Part model, mm, in its own coordinate system. Face numbers are marked on the shaded views. A direction names the side the tool comes from. Round coordinates to 2 decimals unless told otherwise and drop trailing zeros. Order: outer loops, then holes, each group sorted by start corner. A loop starts at its lowest first (then second) coordinate and runs counter-clockwise, first axis right, second up. Notation, with made-up numbers: (61.25, 66.5) - (87.25, 66.5) arc R16 cw to (87.25, 72.5) - close; hole circle Ø8 at (56.25, 64.25). An arc over 180 degrees is marked (long way). Return JSON: item names as keys, results as strings. Group by question number.
Item 1: Saw through at A-A on z = 37.5. List the corners of the cut face in (x, y) (3 decimals).
Item 2: Tool access for the marked faces 1, 2 and 3: list every direction of +Z, -Z, +X, -X, +Y, -Y with a clear straight run to the whole face (end or side of a thin tool).
Item 3: Saw through at D-D on z = 26. List the corners of the cut face in (x, y) (3 decimals), and give its area (3 significant figures).
Item 4: Probe probe 1 along X at (y, z) = (-53, 14.5) (3 decimals); probe 2 along Y at (x, z) = (20, 4.5) (3 decimals); probe 3 along Z at (x, y) = (-15, -66). List the from-to ranges inside material, lowest first.
Item 5: Saw through at C-C on y = -32. List the corners of the cut face in (x, z) (3 decimals), and give its area (3 significant figures).
Item 6: Two-plate mould, pull along X, no slides. Class the marked faces 4, 5, 6 and 7: released by +X, released by -X, zero draft, split by the parting line, or undercut.
Item 7: Drop flat-ended pins along their axis: pin 1 (10 mm diameter, centred on x = -48, y = 30, fed in from -Z); pin 2 (7.5 mm diameter, centred on x = -0.5, y = 6, fed in from +Z); pin 3 (1.5 mm diameter, centred on y = 28.5, z = 28.5, fed in from -X) (3 decimals); pin 4 (1 mm diameter, centred on y = -25, z = 16, fed in from +X) (3 decimals). Give the stop position or say it passes through.
Item 8: Saw through at B-B on x = 45.5. List the corners of the cut face in (y, z) (3 decimals), and give its area (3 significant figures).
```python
from build123d import *

# Parameters (mm, degrees)
F0_W     = 152.5379121304
F0_H     = 152.7792811394
F1_DEPTH = 3.556
F2_W     = 12.7
F2_H     = 50.8
F3_DEPTH = 50.8
F5_DEPTH = 25.4
F6_W     = 61.5432790112
F6_H     = 1.905
F7_DEPTH = 50.8


with BuildPart() as f1:
    # F0 (on Top) → F1 (new body)
    with BuildSketch(Plane.XY):
        with Locations((0.1206770539, 0)):
            Rectangle(F0_W, F0_H)
    extrude(amount=F1_DEPTH)

    # F2 (on face) → F3 (join)
    with BuildSketch(Plane.XY.offset(3.556)):
        with Locations((6.35, 50.9896405697)):
            Rectangle(F2_W, F2_H)
    extrude(amount=F3_DEPTH)

    # F4 (on face) → F5 (cut)
    with BuildSketch(Plane.YZ.offset(12.7)):
        Polygon((25.5896405697, 3.556), (76.3896405697, 54.356), (25.5896405697, 54.356), align=None)
    extrude(amount=-F5_DEPTH, mode=Mode.SUBTRACT)

    # F6 (on face) → F7 (join)
    with BuildSketch(Plane.XY.offset(3.556)):
        with Locations((-45.3766395056, 0.9525)):
            Rectangle(F6_W, F6_H)
        with Locations((-45.3766395056, -0.9525)):
            Rectangle(F6_W, F6_H)
        Polygon((-12.7, 0), (-12.7, 25.5896405697), (-12.7, 76.3896405697), (-14.605, 76.3896405697), (-14.605, 1.905), (-14.605, 0), align=None)
        Polygon((-14.605, -76.3896405697), (-12.7, -76.3896405697), (-12.7, 0), (-14.605, 0), (-14.605, -1.905), align=None)
        Polygon((14.605, 76.3896405697), (12.7, 76.3896405697), (12.7, 25.5896405697), (12.7, 0), (14.605, 0), (14.605, 1.905), align=None)
        Polygon((14.605, 0), (12.7, 0), (12.7, -76.3896405697), (14.605, -76.3896405697), (14.605, -1.905), align=None)
        Polygon((76.1482790112, 1.905), (14.605, 1.905), (14.605, 0), (76.3896331191, 0), (76.3896331191, 1.905), align=None)
        Polygon((76.3896331191, 0), (14.605, 0), (14.605, -1.905), (76.1482790112, -1.905), (76.3896331191, -1.905), align=None)
    extrude(amount=F7_DEPTH)


solid = f1.part
```
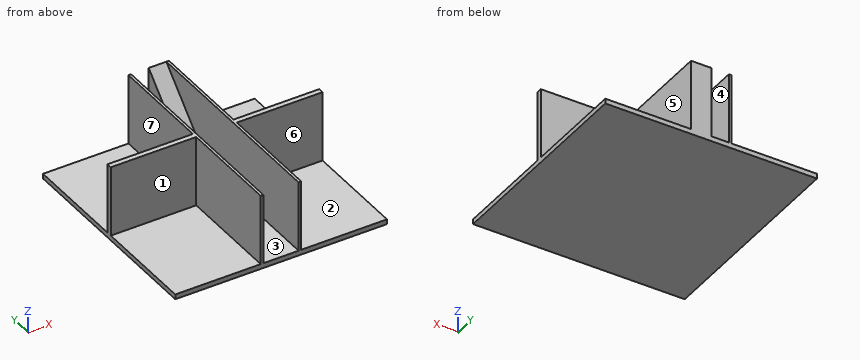
Filled in:
{
 "1": {"outline": "(-76.148, -1.905) - (-14.605, -1.905) - (-14.605, -76.39) - (-12.7, -76.39) - (-12.7, 76.39) - (-14.605, 76.39) - (-14.605, 1.905) - (-76.148, 1.905) - close; (0, 59.534) - (12.7, 59.534) - (12.7, -76.39) - (14.605, -76.39) - (14.605, -1.905) - (76.39, -1.905) - (76.39, 1.905) - (14.605, 1.905) - (14.605, 76.39) - (0, 76.39) - close"},
 "2": {"face 1": "+Z, -X, -Y", "face 2": "+Z, +X, -Y", "face 3": "+Z, -Y"},
 "3": {"outline": "(-76.148, -1.905) - (-14.605, -1.905) - (-14.605, -76.39) - (-12.7, -76.39) - (-12.7, 76.39) - (-14.605, 76.39) - (-14.605, 1.905) - (-76.148, 1.905) - close; (0, 48.034) - (12.7, 48.034) - (12.7, -76.39) - (14.605, -76.39) - (14.605, -1.905) - (76.39, -1.905) - (76.39, 1.905) - (14.605, 1.905) - (14.605, 76.39) - (0, 76.39) - close", "area": "1,410 mm^2"},
 "4": {"probe 1": "x = -14.605 to -12.7, 12.7 to 14.605", "probe 2": "y = -1.905 to 1.905", "probe 3": "z = 0 to 3.56"},
 "5": {"outline": "(-76.148, 0) - (76.39, 0) - (76.39, 3.556) - (14.605, 3.556) - (14.605, 54.356) - (12.7, 54.356) - (12.7, 3.556) - (-12.7, 3.556) - (-12.7, 54.356) - (-14.605, 54.356) - (-14.605, 3.556) - (-76.148, 3.556) - close", "area": "736 mm^2"},
 "6": {"face 4": "undercut", "face 5": "released by +X", "face 6": "zero draft", "face 7": "released by -X"},
 "7": {"pin 1": "stops at z = 0", "pin 2": "stops at z = 3.56", "pin 3": "stops at x = -14.605", "pin 4": "stops at x = 14.605"},
 "8": {"outline": "(-76.39, 0) - (76.39, 0) - (76.39, 3.556) - (1.905, 3.556) - (1.905, 54.356) - (-1.905, 54.356) - (-1.905, 3.556) - (-76.39, 3.556) - close", "area": "737 mm^2"}
}
